```python
from build123d import *

# Parameters (mm, degrees)
SKETCH1_R                     = 31
BOSS_EXTRUDE1_DEPTH           = 7
FILLET1_R                     = 10
M7_CLEARANCE_HOLE1_AT_2_COUNT = 2
M7_CLEARANCE_HOLE1_AT_2_PITCH = 15


with BuildPart() as part:
    # Sketch1 → Boss-Extrude1 (new body, symmetric)
    with BuildSketch(Plane.XY):
        with BuildLine():
            Line((80, 45), (-80, 45))
            Line((-80, 45), (-80, 30.19235911))
            Line((-80, 30.19235911), (-40, 30.19235911))
            Line((-40, 30.19235911), (-36.83773054, -3.461446031))
            ThreePointArc((-36.83773054, -3.461446031), (0, -37), (36.83773054, -3.461446031))
            Line((36.83773054, -3.461446031), (40, 30.19235911))
            Line((40, 30.19235911), (80, 30.19235911))
            Line((80, 30.19235911), (80, 45))
        make_face()
        Circle(SKETCH1_R, mode=Mode.SUBTRACT)
    extrude(amount=BOSS_EXTRUDE1_DEPTH, both=True)

    # Fillet1
    fillet1_edges = [part.edges().sort_by_distance(p)[0] for p in [
        (-40, 30.19235911, 0),
        (40, 30.19235911, 0),
    ]]
    fillet(fillet1_edges, radius=FILLET1_R)

    # Sketch4 → M7 Clearance Hole1 (revolve, cut)
    with BuildSketch(Plane(origin=(-70, 45, 0), x_dir=(0, 0, 1), z_dir=(1, 0, 0))):
        Polygon((0, 0), (0, 22.033270352), (3.8, 19.75), (3.8, 0), align=None)
    m7_clearance_hole1 = revolve(axis=Axis((-70, 51.35, 0), (0, -1, 0)), mode=Mode.SUBTRACT)

    # M7 Clearance Hole1 at 2: M7 Clearance Hole1 ×2
    with Locations(*[(i * M7_CLEARANCE_HOLE1_AT_2_PITCH, 0, 0) for i in range(1, M7_CLEARANCE_HOLE1_AT_2_COUNT)]):
        add(m7_clearance_hole1, mode=Mode.SUBTRACT)

    # Mirror1: M7 Clearance Hole1 across plane
    add(m7_clearance_hole1.mirror(Plane(origin=(0, 0, 0), x_dir=(0, 0, 1), z_dir=(1, 0, 0))), mode=Mode.SUBTRACT)

    # Mirror1 copy 1 sketch → Mirror1 copy 1 (revolve, cut)
    with BuildSketch(Plane(origin=(55, 45, 0), x_dir=(0, 0, 1), z_dir=(-1, 0, 0))):
        Polygon((0, 0), (0, -22.033270352), (3.8, -19.75), (3.8, 0), align=None)
    revolve(axis=Axis((55, 51.35, 0), (0, 1, 0)), mode=Mode.SUBTRACT)


solid = part.part
```
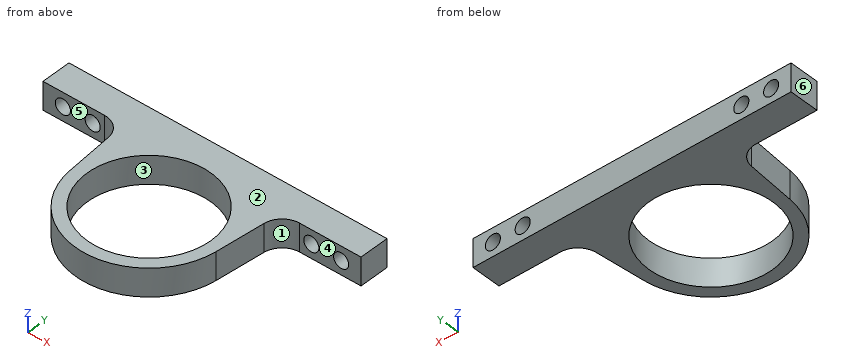
The model under review builds one solid part; all positions refer to its coordinate system, in mm. Face numbers are marked on the shaded views. A direction names the side the tool comes from. Round coordinates to 2 decimals unless told otherwise and drop trailing zeros. Loops run counter-clockwise (first coordinate to the right, second up) from the corner with the lowest first, then second, coordinate; pieces in that order, holes last. Notation, with made-up numbers: M 16.5,27 L 45.5,27 A21 cw 45.5,55 Z; hole C 0.25,66 d9. An arc over 180 degrees is marked long. Put each result on its own line as item: value.
Q1. Consider section C-C, the plane y = -15. Give the boundary of the cut face in (x, z), then the cut area to 3 significant figures.
Result set:
outline: M -33.82,-7 L -27.13,-7 L -27.13,7 L -33.82,7 Z; M 27.13,-7 L 33.82,-7 L 33.82,7 L 27.13,7 Z
area: 187 mm²
Q2. To check wall thickness, follow L1, parallel to X at y = 41, z = 0; L2, parallel to Z at x = -70, y = 37.75; L3, parallel to Y at x = 0, z = -0.25. State the ranges of each line that lie inside material, in increasing order.
Result set:
L1: x = -80 to -73.8, -66.2 to -58.8, -51.2 to 51.2, 58.8 to 66.2, 73.8 to 80
L2: z = -7 to -3.8, 3.8 to 7
L3: y = -37 to -31, 31 to 45
Q3. Mouldability with a two-part tool opening along Y and no side actions: class the marked faces 1, 2 and 3 as released by +Y, released by -Y, zero draft, split by the parting line, or undercut.
Result set:
face 1: released by -Y
face 2: zero draft
face 3: undercut
Q4. For pin 1 (4 mm diameter, centred on x = -16, z = -3, fed in from -Y); pin 2 (6 mm diameter, centred on y = -3.5, z = -2.5, fed in from -X), all flat-tipped, find the tip position at first contact; note any pin that passes through.
Result set:
pin 1: stops at y = -34.25
pin 2: stops at x = -37.12
Q5. Machinability: for the marked faces 4, 5 and 6, which of the approach directions +Z, -Z, +X, -X, +Y, -Y give a long, thin tool a straight path to every point of the face, cutting with its end or side? Answer none if there is none.
Result set:
face 4: +Z, -Z, +X, -Y
face 5: +Z, -Z, -X, -Y
face 6: +Z, -Z, -X, +Y, -Y
Q6. Consider section B-B, the plane x = 70. Give the boundary of the cut face in (y, z), then the cut area to 3 significant figures.
Result set:
outline: M 30.19,-7 L 45,-7 L 45,-3.8 L 30.19,-3.8 Z; M 30.19,3.8 L 45,3.8 L 45,7 L 30.19,7 Z
area: 94.8 mm²
Q7. Consider section A-A, the plane z = 0. Give the boundary of the cut face in (x, y).
Result set:
outline: M -80,30.19 L -73.8,30.19 L -73.8,45 L -80,45 Z; M -66.2,30.19 L -58.8,30.19 L -58.8,45 L -66.2,45 Z; M -51.2,30.19 L -49.1,30.19 A10 cw -39.15,21.13 L -36.84,-3.46 A37 ccw 36.84,-3.46 L 39.15,21.13 A10 cw 49.1,30.19 L 51.2,30.19 L 51.2,45 L -51.2,45 Z; M 58.8,30.19 L 66.2,30.19 L 66.2,45 L 58.8,45 Z; M 73.8,30.19 L 80,30.19 L 80,45 L 73.8,45 Z; hole C 0,0 d62
Q8. Consider section D-D, the plane x = -34. Give the boundary of the cut face in (y, z), then the cut area to 3 significant figures.
Result set:
outline: M -14.59,-7 L 45,-7 L 45,7 L -14.59,7 Z
area: 834 mm²
